For this review, take the finished solid that the model builds, in its own axes (mm). Face numbers are marked on the shaded views. Round coordinates to 2 decimals unless told otherwise and drop trailing zeros. Write each loop counter-clockwise with the first axis right and the second up, starting at its lowest first coordinate (ties: lowest second). Pieces come first, ordered by that corner, then holes. Notation, with made-up numbers: (27, -35) - (40, -35) arc R31 cw to (40, -10) - close; hole circle Ø7 at (18.5, -19.5). An arc over 180 degrees is marked (long way). One line per item, written item: value. Start each with the question number.
Q1. For probe 1 along Y at (x, z) = (2.5, 1.25); probe 2 along Z at (x, y) = (-1.5, 16), list the stretches that pass through material, from the lowest coordinate up.
Q2. Clearance check with flat-ended pins moving along their axes: pin 1 Ø4 at (y, z) = (23.5, 1) entering from +X; pin 2 Ø4.5 at (x, z) = (0, 0) entering from +Y; pin 3 Ø1.5 at (x, y) = (2.5, 15) entering from -Z. State where each tip first meets the part, or that it passes through.
Q3. Add section A-A on y = 23. Write out the cut boundary in (x, z), and give its area (3 significant figures).
Q4. Mouldability with a two-part tool opening along X and no side actions: class the marked faces 1, 2 and 3 as +X half, -X half, draft (parallel to the pull), parting line (faces both ways), or undercut.
```python
from build123d import *

# Parameters (mm, degrees)
SKETCH1_R           = 2.5
BOSS_EXTRUDE1_DEPTH = 29.5
SKETCH2_R           = 3.75
BOSS_EXTRUDE2_DEPTH = 1
SKETCH3_R           = 2
CUT_EXTRUDE2_DEPTH  = 2
FILLET1_R           = 0.5


with BuildPart() as part:
    # Sketch1 → Boss-Extrude1 (new body)
    with BuildSketch(Plane(origin=(0, 0, 0), x_dir=(1, 0, 0), z_dir=(0, 1, 0))):
        with Locations(Location((0, 0, 0), (0, 0, 270))):
            Circle(SKETCH1_R)
    extrude(amount=BOSS_EXTRUDE1_DEPTH)

    # Sketch2 → Boss-Extrude2 (add)
    with BuildSketch(Plane(origin=(0, 29.5, 0), x_dir=(1, 0, 0), z_dir=(0, 1, 0))):
        with Locations(Location((0, 0, 0), (0, 0, 270))):
            Circle(SKETCH2_R)
    extrude(amount=BOSS_EXTRUDE2_DEPTH)

    # Sketch3 → Cut-Extrude2 (cut)
    with BuildSketch(Plane(origin=(0, 30.5, 0), x_dir=(1, 0, 0), z_dir=(0, 1, 0))):
        with Locations(Location((0, 0, 0), (0, 0, 270))):
            Circle(SKETCH3_R)
    extrude(amount=-CUT_EXTRUDE2_DEPTH, mode=Mode.SUBTRACT)

    # Sketch4 → Cut-Revolve1 (revolve, cut)
    with BuildSketch(Plane.XY, mode=Mode.PRIVATE) as cut_revolve1_sk:
        Polygon((-2, 28.5), (0, 26.5), (0, 28.5), align=None)
    revolve(cut_revolve1_sk.sketch.rotate(Axis((0, 26.5, 0), (0, 1, 0)), 90), axis=Axis((0, 26.5, 0), (0, 1, 0)), mode=Mode.SUBTRACT)

    # Fillet1
    fillet1_edges = [part.edges().sort_by_distance(p)[0] for p in [
        (0, 30.5, -2),
        (0, 29.5, -3.75),
        (0, 30.5, -3.75),
    ]]
    fillet(fillet1_edges, radius=FILLET1_R - 0.0001)  # a hair under: the kernel refuses the full size


solid = part.part
```
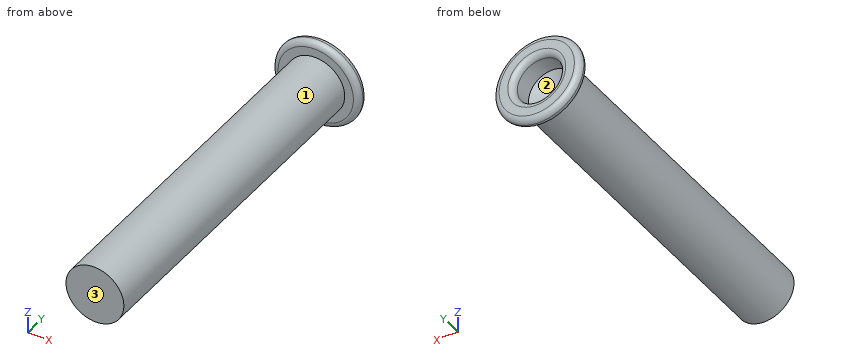
Result set:
1. probe 1: y = 29.5 to 30.5
1. probe 2: z = -2 to 2
2. pin 1: stops at x = 2.5
2. pin 2: stops at y = 30.43
2. pin 3: stops at z = -1.79
3. outline: circle Ø5 at (0, 0)
3. area: 19.6 mm^2
4. face 1: parting line
4. face 2: undercut
4. face 3: draft
